The listing builds one solid part. Answer for the finished solid, in the listing's coordinates (mm). A direction names the side the tool comes from. Round coordinates to 2 decimals unless told otherwise and drop trailing zeros. Write each loop counter-clockwise with the first axis right and the second up, starting at its lowest first coordinate (ties: lowest second). Pieces come first, ordered by that corner, then holes. Notation, with made-up numbers: M 89,-16.5 L 123,-16.5 A29 cw 123,17.5 Z; hole C 81,36 d6. An arc over 180 degrees is marked long. Put each result on its own line as item: value. Start each with the question number.
```python
from build123d import *

# Parameters (mm, degrees)
CROQUIS1_W              = 20
CROQUIS1_H              = 16.5
SALIENTE_EXTRUIR1_DEPTH = 3.3
CROQUIS2_W              = 1.4
CROQUIS2_H              = 3.7
SALIENTE_EXTRUIR2_DEPTH = 1.4
CORTAR_EXTRUIR1_DEPTH   = 3.7
CORTAR_EXTRUIR2_DEPTH   = 3.7
CROQUIS6_W              = 20
CROQUIS6_H              = 16.5
SALIENTE_EXTRUIR3_DEPTH = 3.3
CROQUIS7_W              = 1.4
CROQUIS7_H              = 3.7
SALIENTE_EXTRUIR4_DEPTH = 1.4
CORTAR_EXTRUIR3_DEPTH   = 3.7
CORTAR_EXTRUIR4_DEPTH   = 3.7
SALIENTE_EXTRUIR5_DEPTH = 2.2
SALIENTE_EXTRUIR6_DEPTH = 2.2


with BuildPart() as part:
    # Croquis1 → Saliente-Extruir1 (new body)
    with BuildSketch(Plane.XY):
        Rectangle(CROQUIS1_W, CROQUIS1_H)
        with BuildLine():
            Line((-1.55, 3), (1.55, 3))
            ThreePointArc((1.55, 3), (4.55, 0), (1.55, -3))
            Line((1.55, -3), (-1.55, -3))
            ThreePointArc((-1.55, -3), (-4.55, 0), (-1.55, 3))
        make_face(mode=Mode.SUBTRACT)
    extrude(amount=SALIENTE_EXTRUIR1_DEPTH)

    # Croquis2 → Saliente-Extruir2 (add)
    with BuildSketch(Plane.XY.offset(3.3)):
        with Locations((-7.5, 0)):
            Rectangle(CROQUIS2_W, CROQUIS2_H)
        with Locations((7.5, 0)):
            Rectangle(CROQUIS2_W, CROQUIS2_H)
    extrude(amount=SALIENTE_EXTRUIR2_DEPTH)

    # Croquis4 → Cortar-Extruir1 (cut)
    with BuildSketch(Plane.XZ.offset(1.85)):
        Polygon((8.2, 3.3), (7.6, 4.7), (8.2, 4.7), align=None)
    extrude(amount=-CORTAR_EXTRUIR1_DEPTH, mode=Mode.SUBTRACT)

    # Croquis5 → Cortar-Extruir2 (cut)
    with BuildSketch(Plane.XZ.offset(1.85)):
        Polygon((-6.8, 3.3), (-7.4, 4.7), (-6.8, 4.7), align=None)
    extrude(amount=-CORTAR_EXTRUIR2_DEPTH, mode=Mode.SUBTRACT)

    # Croquis6 → Saliente-Extruir3 (add)
    with BuildSketch(Plane(origin=(10, 0, 0), x_dir=(0, 0, -1), z_dir=(1, 0, 0))):
        with Locations((6.7, 0)):
            Rectangle(CROQUIS6_W, CROQUIS6_H)
        with BuildLine():
            Line((5.15, 3), (8.25, 3))
            ThreePointArc((8.25, 3), (11.25, 0), (8.25, -3))
            Line((8.25, -3), (5.15, -3))
            ThreePointArc((5.15, -3), (2.15, 0), (5.15, 3))
        make_face(mode=Mode.SUBTRACT)
    extrude(amount=-SALIENTE_EXTRUIR3_DEPTH)

    # Croquis7 → Saliente-Extruir4 (add)
    with BuildSketch(Plane(origin=(10, 0, 0), x_dir=(0, 0, -1), z_dir=(1, 0, 0))):
        with Locations((-0.8, 0)):
            Rectangle(CROQUIS7_W, CROQUIS7_H)
        with Locations((14.2, 0)):
            Rectangle(CROQUIS7_W, CROQUIS7_H)
    extrude(amount=SALIENTE_EXTRUIR4_DEPTH)

    # Croquis11 → Cortar-Extruir3 (cut)
    with BuildSketch(Plane.XZ.offset(1.85)):
        Polygon((11.4, 0.1), (10, 0.1), (11.4, 0.7), align=None)
    extrude(amount=-CORTAR_EXTRUIR3_DEPTH, mode=Mode.SUBTRACT)

    # Croquis12 → Cortar-Extruir4 (cut)
    with BuildSketch(Plane.XZ.offset(1.85)):
        Polygon((11.4, -14.9), (10, -14.9), (11.4, -14.3), align=None)
    extrude(amount=-CORTAR_EXTRUIR4_DEPTH, mode=Mode.SUBTRACT)

    # Croquis13 → Saliente-Extruir5 (add)
    with BuildSketch(Plane(origin=(0, -8.25, 0), x_dir=(-1, 0, 0), z_dir=(0, -1, 0))):
        Polygon((-6.7, 16.7), (10, 0), (-6.7, 0), align=None)
    extrude(amount=-SALIENTE_EXTRUIR5_DEPTH)

    # Croquis14 → Saliente-Extruir6 (add)
    with BuildSketch(Plane(origin=(0, 8.25, 0), x_dir=(1, 0, 0), z_dir=(0, 1, 0))):
        Polygon((6.7, 16.7), (-10, 0), (6.7, 0), align=None)
    extrude(amount=-SALIENTE_EXTRUIR6_DEPTH)


solid = part.part
```
Item 1: Section C-C (x = -6.25) is taken. Give the vertices of the cut face in (y, z), and give its area (4 significant figures).
Item 2: Consider line 1 along Y through (x, z) = (-5.75, -1); line 2 along Z through (x, y) = (-3.5, 4.75); line 3 along X through (y, z) = (-7.5, 1). Determine where each line is inside the solid, lowest interval first. Write a range as [from, to].
Item 3: Flat-ended cylindrical pins translate along their axes: pin 1 (0.7 mm diameter, centred on x = 10.5, z = 0.5, fed in from +Y); pin 2 (0.7 mm diameter, centred on y = 0, z = 4, fed in from -X); pin 3 (2 mm diameter, centred on x = 3.5, y = 3.5, fed in from -Z). Find the tip coordinate at first contact, or state that the pin passes through.
Item 4: Section D-D (z = -4.25) is taken. Give the vertices of the cut face in (x, y), and give its area (3 significant figures).
Item 5: Section B-B (y = 0) is taken. Count the separate pieces of the cut face and the enclosed holes in it, and give its area (3 significant figures).
Item 6: Section A-A (z = 2.5) is taken. Give the vertices of the cut face in (x, y), and give its area (3 significant figures).
Item 7: Determine the mould class of faces 1 (the cylindrical face through (8.37, -0.07, -2.15)), 2 (the flat face through (2, 8.25, -5)), 3 (the flat face through (-2, 7, -8)), 4 (the flat face through (-7.1, 0, 4)) for opening direction Z: released by +Z, released by -Z, zero draft, split by the parting line, or undercut.
Item 8: Which of the six approach directions +Z, -Z, +X, -X, +Y, -Y give full straight-line access (tool end or side, diameter ignored) to faces 5 (the cylindrical face through (-4.55, -0.07, 1.63)), 6 (the flat face through (2, 6.05, -5)), 7 (the flat face through (-8, -1.85, 4)), 8 (the flat face through (8, -3, -7))?
Output values:
1. outline: M -8.25,-3.75 L -6.05,-3.75 L -6.05,0 L 6.05,0 L 6.05,-3.75 L 8.25,-3.75 L 8.25,3.3 L -8.25,3.3 Z
1. area: 70.95 mm^2
2. line 1: y = [-8.25, -6.05], [6.05, 8.25]
2. line 2: z = [0, 3.3]
2. line 3: x = [-10, 10]
3. pin 1: stops at y = 1.85
3. pin 2: stops at x = -8.2
3. pin 3: stops at z = 0
4. outline: M -5.75,-8.25 L 10,-8.25 L 10,-2.86 L 6.7,-2.86 L 6.7,-6.05 L -5.75,-6.05 Z; M -5.75,6.05 L 6.7,6.05 L 6.7,2.86 L 10,2.86 L 10,8.25 L -5.75,8.25 Z
4. area: 90.3 mm^2
5. separate pieces: 3
5. enclosed holes: 0
5. area: 67.2 mm^2
6. outline: M -10,-8.25 L 10,-8.25 L 10,8.25 L -10,8.25 Z; hole M -1.55,-3 L 1.55,-3 A3 ccw 1.55,3 L -1.55,3 A3 ccw Z
6. area: 283 mm^2
7. face 1: undercut
7. face 2: zero draft
7. face 3: released by -Z
7. face 4: released by +Z
8. face 5: +Z, -Z
8. face 6: -Z, -X
8. face 7: +Z, +X, -X, -Y
8. face 8: +X, -X
